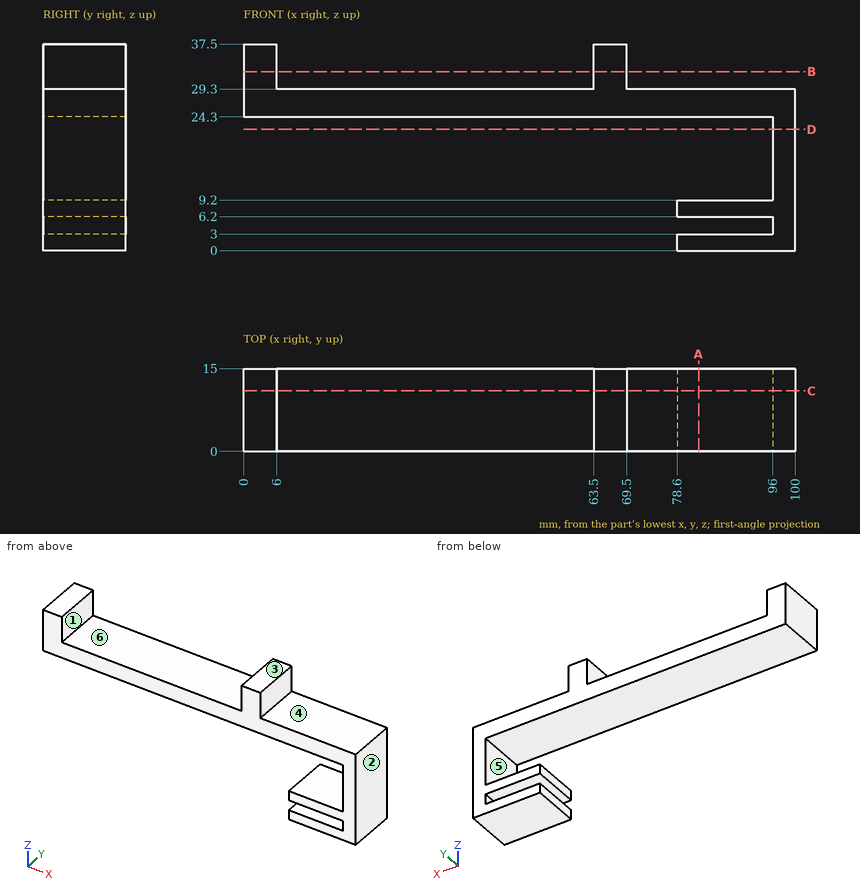
Can you work these out from the drawing? Everything is in mm from the part's minimum corner. A direction names the side the tool comes from. Coordinates: 2 decimals unless noted, no trailing zeros. Loops run counter-clockwise (first coordinate to the right, second up) from the corner with the lowest first, then second, coordinate; pieces in that order, holes last.
1) Imagine slicing it at C-C (y = 11). List the corners of the cut face in (x, z) for me, and give its area (3 significant figures).
Reported:
outline: (0, 24.3) - (96, 24.3) - (96, 9.2) - (78.6, 9.2) - (78.6, 6.2) - (96, 6.2) - (96, 3) - (78.6, 3) - (78.6, 0) - (100, 0) - (100, 29.3) - (69.5, 29.3) - (69.5, 37.5) - (63.5, 37.5) - (63.5, 29.3) - (6, 29.3) - (6, 37.5) - (0, 37.5) - close
area: 800 mm2
2) Imagine slicing it at A-A (x = 82.5). List the corners of the cut face in (y, z) for me.
Reported:
outline: (0, 0) - (15, 0) - (15, 3) - (0, 3) - close; (0, 6.2) - (15, 6.2) - (15, 9.2) - (0, 9.2) - close; (0, 24.3) - (15, 24.3) - (15, 29.3) - (0, 29.3) - close
3) Imagine slicing it at B-B (z = 32.5). List the corners of the cut face in (x, y) for me.
Reported:
outline: (0, 0) - (6, 0) - (6, 15) - (0, 15) - close; (63.5, 0) - (69.5, 0) - (69.5, 15) - (63.5, 15) - close
4) Which directions (+Z, -Z, +X, -X, +Y, -Y) give clear straight access to the entire face, cutting with the end or side of a thin tool? Please do the marked faces 4, 5 and 6.
Reported:
face 4: +Z, +X, +Y, -Y
face 5: -X, +Y, -Y
face 6: +Z, +Y, -Y
5) Thinking about a two-plate mould opening in X: for the marked faces 1, 2 and 3, which applies, released by +X, released by -X, zero draft, split by the parting line, or undercut?
Reported:
face 1: undercut
face 2: released by +X
face 3: zero draft
6) Imagine slicing it at D-D (z = 22). List the corners of the cut face in (x, y) for me, and give its area (3 significant figures).
Reported:
outline: (96, 0) - (100, 0) - (100, 15) - (96, 15) - close
area: 60.0 mm2
7) Please list where these lines run through material, in increasing order: line 1 along X through (y, z) = (11, 33); line 2 along Z through (x, y) = (35, 9.25); line 3 along X through (y, z) = (8.25, 11).
Reported:
line 1: x = 0 to 6, 63.5 to 69.5
line 2: z = 24.3 to 29.3
line 3: x = 96 to 100
8) Will these pins go through, and if not, where does the flat tip stop? pin 1 Ø7.5 at (x, y) = (89, 6) entering from +Z; pin 2 Ø4.5 at (y, z) = (7, 19) entering from -X; pin 3 Ø0.9 at (y, z) = (10.5, 2) entering from -X.
Reported:
pin 1: stops at z = 29.3
pin 2: stops at x = 96
pin 3: stops at x = 78.6
